Verification items for the finished model (mm, model axes). A direction names the side the tool comes from. Coordinates: 2 decimals unless noted, no trailing zeros. Order: outer loops, then holes, each group sorted by start corner. A loop starts at its lowest first (then second) coordinate and runs counter-clockwise, first axis right, second up. Notation, with made-up numbers: M -35,34 L 8,34 A31 ccw 8,60 Z; hole C -2.5,25.5 d2. An arc over 180 degrees is marked long. Answer as a JSON object with one key per item and string values. Group by question number.
(1) Cross-section at B-B (y = 0). Enter the section's corners in (x, z) (3 decimals), plus the area to 3 significant figures.
(2) Cross-section at C-C (z = -75). Enter the section's corners in (x, y), plus the area to 3 significant figures.
(3) Material ranges on line 1 (X direction, y = 4.5, z = 16.5) (3 decimals); line 2 (Z direction, x = -11, y = -6.25) (3 decimals); line 3 (Z direction, x = -7, y = -3.75) (3 decimals), recorded low to high.
(4) Gauge pin test, flat ends, axial feed: pin 1 Ø1.5 at (y, z) = (-6, -47.5) entering from -X; pin 2 Ø10 at (x, y) = (31, 9) entering from -Z; pin 3 Ø10 at (x, y) = (10, 5.5) entering from -Z. Record the tip position at first contact, or that the pin passes through.
(5) Mould release check, pull along X, two halves, no side actions. Record for faces 1 (the face through (-41.275, 0, 11)), 2 (the face through (-5, 9, -12.7)), 3 (the face through (9.525, 0, 16)), 4 (the face through (12.7, 0, -6)): released by +X, released by -X, zero draft, split by the parting line, or undercut.
(6) Cross-section at A-A (x = 0). Enter the section's corners in (y, z) (3 decimals), plus the area to 3 significant figures.
(7) Access from +Z, -Z, +X, -X, +Y, -Y to the whole of each face (thin tool, end or side, straight path). Record for faces 5 (the face through (41.275, 0, 11)), 6 (the face through (2, 6.2, -38.1)), 7 (the face through (-12.7, 0, -6)), 8 (the face through (27, 0, 0)), 9 (the face through (0, 0, 9.525)).
(8) Cross-section at D-D (z = -20.5). Enter the section's corners in (x, y) (3 decimals).
from build123d import *

# Parameters (mm, degrees)
BOSS_EXTRUDE1_DEPTH = 12.7
SKETCH2_R           = 9.525
BOSS_EXTRUDE2_DEPTH = 25.4
SKETCH3_R           = 6.35
BOSS_EXTRUDE3_DEPTH = 76.2


with BuildPart() as part:
    # Sketch1 → Boss-Extrude1 (new, symmetric)
    with BuildSketch(Plane(origin=(0, 0, 0), x_dir=(1, 0, 0), z_dir=(0, 1, 0))):
        Polygon((12.7, 12.7), (-12.7, 12.7), (-12.7, 0), (-41.275, 0), (-41.275, -22.225), (-9.525, -22.225), (-9.525, -9.525), (9.525, -9.525), (9.525, -22.225), (41.275, -22.225), (41.275, 0), (12.7, 0), align=None)
    extrude(amount=BOSS_EXTRUDE1_DEPTH, both=True)

    # Sketch2 → Boss-Extrude2 (add)
    with BuildSketch(Plane(origin=(0, 0, -12.7), x_dir=(-1, 0, 0), z_dir=(0, 0, -1))):
        with Locations(Location((0, 0, 0), (0, 0, 180))):
            Circle(SKETCH2_R)
    extrude(amount=BOSS_EXTRUDE2_DEPTH)

    # Sketch3 → Boss-Extrude3 (add)
    with BuildSketch(Plane(origin=(0, 0, -38.1), x_dir=(-1, 0, 0), z_dir=(0, 0, -1))):
        with Locations(Location((0, 0, 0), (0, 0, 180))):
            Circle(SKETCH3_R)
    extrude(amount=BOSS_EXTRUDE3_DEPTH)


solid = part.part
Taken from the geometry:
{
 "1": {"outline": "M -41.275,0 L -12.7,0 L -12.7,-12.7 L -9.525,-12.7 L -9.525,-38.1 L -6.35,-38.1 L -6.35,-114.3 L 6.35,-114.3 L 6.35,-38.1 L 9.525,-38.1 L 9.525,-12.7 L 12.7,-12.7 L 12.7,0 L 41.275,0 L 41.275,22.225 L 9.525,22.225 L 9.525,9.525 L -9.525,9.525 L -9.525,22.225 L -41.275,22.225 Z", "area": "3,370 mm²"},
 "2": {"outline": "C 0,0 d12.7", "area": "127 mm²"},
 "3": {"line 1": "x = -41.275 to -9.525, 9.525 to 41.275", "line 2": "z = -12.7 to 22.225", "line 3": "z = -38.1 to 9.525"},
 "4": {"pin 1": "stops at x = -3.57", "pin 2": "stops at z = 0", "pin 3": "stops at z = -38.1"},
 "5": {"face 1": "released by -X", "face 2": "zero draft", "face 3": "undercut", "face 4": "released by +X"},
 "6": {"outline": "M -12.7,-12.7 L -9.525,-12.7 L -9.525,-38.1 L -6.35,-38.1 L -6.35,-114.3 L 6.35,-114.3 L 6.35,-38.1 L 9.525,-38.1 L 9.525,-12.7 L 12.7,-12.7 L 12.7,9.525 L -12.7,9.525 Z", "area": "2,020 mm²"},
 "7": {"face 5": "+Z, -Z, +X, +Y, -Y", "face 6": "-Z", "face 7": "-Z, -X, +Y, -Y", "face 8": "-Z, +X, +Y, -Y", "face 9": "+Z, +Y, -Y"},
 "8": {"outline": "C 0,0 d19.05"}
}
